```python
from build123d import *

# Parameters (mm, degrees)
SKETCH_1_W          = 70
SKETCH_1_H          = 70
EXTRUDE_1_DEPTH     = 2.2
SKETCH_2_W          = 30
SKETCH_2_H          = 30
CUT_EXTRUDE_1_DEPTH = 1.4
SKETCH_3_R          = 2.6
CUT_EXTRUDE_2_DEPTH = 3.2
EXTRUDE_2_DEPTH     = 1.8
SKETCH_6_R          = 1.6
EXTRUDE_3_DEPTH     = 0.3


with BuildPart() as part:
    # 草图1 → 凸台-拉伸1 (new body)
    with BuildSketch(Plane.XY):
        with BuildLine():
            Line((-2, 17), (0, 17))
            Line((0, 17), (0, 53))
            Line((0, 53), (-2, 53))
            ThreePointArc((-2, 53), (-4.121320344, 52.121320344), (-5, 50))
            Line((-5, 50), (-5, 20))
            ThreePointArc((-5, 20), (-4.121320344, 17.878679656), (-2, 17))
        make_face()
        with Locations((35, 35)):
            Rectangle(SKETCH_1_W, SKETCH_1_H)
        with BuildLine():
            Line((70, 53), (70, 17))
            Line((70, 17), (72, 17))
            ThreePointArc((72, 17), (74.121320344, 17.878679656), (75, 20))
            Line((75, 20), (75, 50))
            ThreePointArc((75, 50), (74.121320344, 52.121320344), (72, 53))
            Line((72, 53), (70, 53))
        make_face()
    extrude(amount=EXTRUDE_1_DEPTH)

    # 草图2 → 切除-拉伸1 (cut)
    with BuildSketch(Plane.XY.offset(2.2)):
        with Locations((35, 35)):
            Rectangle(SKETCH_2_W, SKETCH_2_H)
    extrude(amount=-CUT_EXTRUDE_1_DEPTH, mode=Mode.SUBTRACT)

    # 草图3 → 切除-拉伸2 (cut, through all)
    with BuildSketch(Plane.XY.offset(2.2)):
        with Locations((8, 62)):
            Circle(SKETCH_3_R)
        with Locations((62, 62)):
            Circle(SKETCH_3_R)
        with Locations((8, 8)):
            Circle(SKETCH_3_R)
        with Locations((62, 8)):
            Circle(SKETCH_3_R)
    extrude(amount=-CUT_EXTRUDE_2_DEPTH, mode=Mode.SUBTRACT)

    # 草图4 → 凸台-拉伸2 (add)
    with BuildSketch(Plane.XY):
        with BuildLine():
            Line((20, 44), (20, 50))
            Line((20, 50), (26, 50))
            ThreePointArc((26, 50), (24.242640687, 45.757359313), (20, 44))
        make_face()
        with BuildLine():
            Line((50, 44), (50, 50))
            Line((50, 50), (44, 50))
            ThreePointArc((44, 50), (45.757359313, 45.757359313), (50, 44))
        make_face()
        with BuildLine():
            Line((50, 20), (44, 20))
            ThreePointArc((44, 20), (45.757359313, 24.242640687), (50, 26))
            Line((50, 26), (50, 20))
        make_face()
        with BuildLine():
            Line((20, 26), (20, 20))
            Line((20, 20), (26, 20))
            ThreePointArc((26, 20), (24.242640687, 24.242640687), (20, 26))
        make_face()
    extrude(amount=EXTRUDE_2_DEPTH)

    # 草图6 → 凸台-拉伸3 (add)
    with BuildSketch(Plane.XY.offset(1.8)):
        with Locations((22.5, 47.5)):
            Circle(SKETCH_6_R)
        with Locations((47.5, 47.5)):
            Circle(SKETCH_6_R)
        with Locations((47.5, 22.5)):
            Circle(SKETCH_6_R)
        with Locations((22.5, 22.5)):
            Circle(SKETCH_6_R)
        Polygon((20.1, 45.5), (20.7, 45.5), (20.7, 46.1), (21.3, 46.1), (21.3, 45.5), (21.9, 45.5), (21.9, 44.9), (21.3, 44.9), (21.3, 44.3), (20.7, 44.3), (20.7, 44.9), (20.1, 44.9), align=None)
    extrude(amount=EXTRUDE_3_DEPTH)


solid = part.part
```
Design review of the part built by this model. Coordinates are the model's own, in mm. A direction names the side the tool comes from. Give positions to 0.01 mm unless a question says otherwise; leave off trailing zeros. Order: outer loops, then holes, each group sorted by start corner. A loop starts at its lowest first (then second) coordinate and runs counter-clockwise, first axis right, second up. Notation, with made-up numbers: (78, -13) - (100, -13) arc R35 ccw to (100, 22) - close; hole circle Ø9 at (38, 85.25). An arc over 180 degrees is marked (long way). Use a Markdown table: item, result. Add a question column.
(1) Add section D-D on y = 38.5. Give the boundary of the cut face in (x, z), then the cut area to 3 significant figures.
(2) Add section C-C on x = 40. Give the boundary of the cut face in (y, z).
(3) Clearance check with flat-ended pins moving along their axes: P1, Ø3.5, axis at x = 22.5, y = 48, coming from the +Z side; P2, Ø1, axis at y = 14.5, z = 1.5, coming from the -X side; P3, Ø15, axis at x = 35.5, y = 39.5, coming from the +Z side. State where each tip first meets the part, or that it passes through.
(4) Add section A-A on x = 61. Give the boundary of the cut face in (y, z).
(5) Add section B-B on y = 8. Give the boundary of the cut face in (x, z).
(6) Wall thickness on probe 1 along Y at (x, z) = (62, 0.5); probe 2 along Y at (x, z) = (32.5, 1.3); probe 3 along Y at (x, z) = (6.5, 1.9): over which ranges is each line inside the solid? List them lowest first. Write a range as [from, to].
(7) Machinability: for faces 1 (the face through (0, 61, 1)), 2 (the face through (-5, 35, 1)), 3 (the face through (70, 8, 1)), 4 (the face through (-4.14, 17.9, 1.08)), 5 (the face through (22, 48, 2.1)), which of the approach directions +Z, -Z, +X, -X, +Y, -Y give a long, thin tool a straight path to every point of the face, cutting with its end or side? Answer none if there is none.
(8) Mouldability with a two-part tool opening along Y and no side actions: class faces 6 (the face through (71, 17, 1)), 7 (the face through (35, 70, 1)), 8 (the face through (21, 45, 2.1)) as +Y half, -Y half, draft (parallel to the pull), parting line (faces both ways), or undercut.
Report:
| question | item | result |
|---|---|---|
| 1 | outline | (-5, 0) - (75, 0) - (75, 2.2) - (50, 2.2) - (50, 0.8) - (20, 0.8) - (20, 2.2) - (-5, 2.2) - close |
| 1 | area | 134 mm² |
| 2 | outline | (0, 0) - (70, 0) - (70, 2.2) - (50, 2.2) - (50, 0.8) - (20, 0.8) - (20, 2.2) - (0, 2.2) - close |
| 3 | P1 | stops at z = 2.1 |
| 3 | P2 | stops at x = 0 |
| 3 | P3 | stops at z = 0.8 |
| 4 | outline | (0, 0) - (5.6, 0) - (5.6, 2.2) - (0, 2.2) - close; (10.4, 0) - (59.6, 0) - (59.6, 2.2) - (10.4, 2.2) - close; (64.4, 0) - (70, 0) - (70, 2.2) - (64.4, 2.2) - close |
| 5 | outline | (0, 0) - (5.4, 0) - (5.4, 2.2) - (0, 2.2) - close; (10.6, 0) - (59.4, 0) - (59.4, 2.2) - (10.6, 2.2) - close; (64.6, 0) - (70, 0) - (70, 2.2) - (64.6, 2.2) - close |
| 6 | probe 1 | y = [0, 5.4], [10.6, 59.4], [64.6, 70] |
| 6 | probe 2 | y = [0, 20], [50, 70] |
| 6 | probe 3 | y = [0, 5.88], [10.12, 59.88], [64.12, 70] |
| 7 | face 1 | +Z, -Z, -X, +Y |
| 7 | face 2 | +Z, -Z, -X, +Y, -Y |
| 7 | face 3 | +Z, -Z, +X, -Y |
| 7 | face 4 | +Z, -Z, -X, -Y |
| 7 | face 5 | +Z |
| 8 | face 6 | -Y half |
| 8 | face 7 | +Y half |
| 8 | face 8 | undercut |
